Could you check a few things on this model? Use its own coordinates, in mm. A direction names the side the tool comes from. Round coordinates to 2 decimals unless told otherwise and drop trailing zeros. Loops run counter-clockwise (first coordinate to the right, second up) from the corner with the lowest first, then second, coordinate; pieces in that order, holes last. Notation, with made-up numbers: M 33.25,-33.5 L 39.25,-33.5 A13 cw 39.25,-18.5 Z; hole C 58.25,-40 d7. An arc over 180 degrees is marked long. Answer in a Markdown table with one row per item.
```python
from build123d import *

# Parameters (mm, degrees)
F1_DEPTH = 50
F2_T     = 1
F4_D     = 30
F5_D     = 20
F6_D     = 25
F7_D     = 10
F8_D     = 5
F9_D     = 15


with BuildPart() as f1:
    # F0 (on Top) → F1 (new body)
    with BuildSketch(Plane.XY):
        Polygon((-20.9249958888, -14.6793369754), (-20.9249958888, 127.5117987929), (-59.0249958888, -14.6793369754), align=None)
    extrude(amount=F1_DEPTH)

    # F2
    f2_openings = [f1.faces().sort_by_distance(p)[0] for p in [
        (-33.624996, 32.717708, 50),
    ]]
    offset(amount=F2_T, openings=f2_openings, kind=Kind.INTERSECTION)

    # F4 (through all)
    with Locations(Plane.YZ.offset(-19.9249958888)):
        with Locations((114.3206630246, 24.5)):
            Hole(F4_D / 2)

    # F5 (through all)
    with Locations(Plane.YZ.offset(-19.9249958888)):
        with Locations((-0.6793369754, 24.5)):
            Hole(F5_D / 2)

    # F6 (through all)
    with Locations(Plane.YZ.offset(-19.9249958888)):
        with Locations((45.3206630246, 24.5)):
            Hole(F6_D / 2)

    # F7 (through all)
    with Locations(Plane.YZ.offset(-19.9249958888)):
        with Locations((68.3206630246, 24.5)):
            Hole(F7_D / 2)

    # F8 (through all)
    with Locations(Plane.YZ.offset(-19.9249958888)):
        with Locations((91.3206630246, 24.5)):
            Hole(F8_D / 2)

    # F9 (through all)
    with Locations(Plane.YZ.offset(-19.9249958888)):
        with Locations((22.3206630246, 24.5)):
            Hole(F9_D / 2)


solid = f1.part
```
1) I want a section at A-A, the plane y = 27. Please give me the cut outline in (x, z) (3 decimals).
Computed:
| item | result |
|---|---|
| outline | M -48.892,-1 L -19.925,-1 L -19.925,18.639 L -20.925,18.639 L -20.925,0 L -47.857,0 L -47.857,18.639 L -48.892,18.639 Z; M -48.892,30.361 L -47.857,30.361 L -47.857,50 L -48.892,50 Z; M -20.925,30.361 L -19.925,30.361 L -19.925,50 L -20.925,50 Z |
2) I want a section at C-C, the plane z = 24.5. State how many separate pieces and enclosed holes the cut face has, plus the area to 3 significant figures.
Computed:
| item | result |
|---|---|
| separate pieces | 12 |
| enclosed holes | 0 |
| area | 124 mm² |
3) Which directions (+Z, -Z, +X, -X, +Y, -Y) give clear straight access to the entire face, cutting with the end or side of a thin tool? Please do faces 4 (the face through (-32, 26, 0)), 5 (the face through (-20.432, 69.405, 19.619)).
Computed:
| item | result |
|---|---|
| face 4 | +Z |
| face 5 | +X, -X |
4) I need wall thicknesses on line 1 (Z direction, x = -22, y = 111); line 2 (X direction, y = 29.5, z = 41.5) (3 decimals); line 3 (X direction, y = 57.5, z = 14.5) (3 decimals). Which ranges of each line are inside material? Lowest first, please.
Computed:
| item | result |
|---|---|
| line 1 | z = -1 to 0 |
| line 2 | x = -48.222 to -47.187, -20.925 to -19.925 |
| line 3 | x = -40.72 to -39.685, -20.925 to -19.925 |
5) I want a section at B-B, the plane y = 5.5. Please give me the cut outline in (x, z) (3 decimals), plus the area to 3 significant figures.
Computed:
| item | result |
|---|---|
| outline | M -54.653,-1 L -19.925,-1 L -19.925,16.638 L -20.925,16.638 L -20.925,0 L -53.618,0 L -53.618,16.638 L -54.653,16.638 Z; M -54.653,32.362 L -53.618,32.362 L -53.618,50 L -54.653,50 Z; M -20.925,32.362 L -19.925,32.362 L -19.925,50 L -20.925,50 Z |
| area | 104 mm² |
6) Will these pins go through, and if not, where does the flat tip stop? P1, Ø8, axis at x = -38.5, y = 67.5, coming from the +Z side; P2, Ø8, axis at y = 30.5, z = 18, coming from the -X side; P3, Ø4, axis at y = 102, z = 42, coming from the -X side; P4, Ø1, axis at y = 19.5, z = 15, coming from the -X side.
Computed:
| item | result |
|---|---|
| P1 | stops at z = 50 |
| P2 | stops at x = -49.03 |
| P3 | stops at x = -29.33 |
| P4 | stops at x = -51.04 |
7) If we mould it in two halves opening along Y, with no side actions, what happens to faces 1 (the face through (-39.844, 60.77, 24.143)), 2 (the face through (-20.925, 55, 36)), 3 (the face through (-40, -15.679, 24))? For each: released by +Y, released by -Y, zero draft, split by the parting line, or undercut.
Computed:
| item | result |
|---|---|
| face 1 | released by +Y |
| face 2 | undercut |
| face 3 | released by -Y |
